The listing builds one solid part. Answer for the finished solid, in the listing's coordinates (mm). Round coordinates to 2 decimals unless told otherwise and drop trailing zeros. Loops run counter-clockwise (first coordinate to the right, second up) from the corner with the lowest first, then second, coordinate; pieces in that order, holes last. Notation, with made-up numbers: (84.25, -12) -> (93.25, -12) arc R13 ccw to (93.25, -7) -> close; hole circle Ø2 at (76.25, 71). An arc over 180 degrees is marked (long way). One line per question, with ' | ' between items.
from build123d import *

# Parameters (mm, degrees)
SKETCH1_R           = 5.56895
BOSS_EXTRUDE1_DEPTH = 23.8125
SKETCH2_R           = 1.5875
BOSS_EXTRUDE2_DEPTH = 3.175


with BuildPart() as part:
    # Sketch1 → Boss-Extrude1 (new, symmetric)
    with BuildSketch(Plane(origin=(0, 0, 0), x_dir=(0, 0, -1), z_dir=(1, 0, 0))):
        Circle(SKETCH1_R)
    extrude(amount=BOSS_EXTRUDE1_DEPTH, both=True)

    # Sketch2 → Boss-Extrude2 (add)
    with BuildSketch(Plane.ZY.offset(23.8125)):
        Circle(SKETCH2_R)
    boss_extrude2 = extrude(amount=BOSS_EXTRUDE2_DEPTH)

    # Sketch5 → Revolve1 (revolve)
    with BuildSketch(Plane.XY):
        with BuildLine():
            Line((-35.1917, 0), (-26.3525, 0))
            ThreePointArc((-26.3525, 0), (-30.7721, 4.4196), (-35.1917, 0))
        make_face()
    revolve1 = revolve(axis=Axis((-35.1917, 0, 0), (1, 0, 0)))

    # Mirror2: Boss-Extrude2, Revolve1 across plane
    add(boss_extrude2.mirror(Plane(origin=(0, 0, 0), x_dir=(0, 0, 1), z_dir=(1, 0, 0))))
    add(revolve1.mirror(Plane(origin=(0, 0, 0), x_dir=(0, 0, 1), z_dir=(1, 0, 0))))


solid = part.part
Q1. For a pull along X with two mould halves and no side action, classify faces 1 (the face through (0.333, 5.522, 0.725)), 2 (the face through (-23.812, 1.3, -1.2)), 3 (the face through (25.21, 0.477, 1.514)) as pulls with the +X half, pulls with the -X half, needs draft (parallel to the pull), parting line crosses it, or undercut.
Numbers:
face 1: needs draft | face 2: undercut | face 3: undercut
Q2. A cutting plane is placed at A-A on y = 0. Give the vertices of the cut face in (x, z).
Numbers:
outline: (-26.65, -1.59) -> (-23.81, -1.59) -> (-23.81, -5.57) -> (23.81, -5.57) -> (23.81, -1.59) -> (26.65, -1.59) arc R4.42 ccw (long way) to (26.65, 1.59) -> (23.81, 1.59) -> (23.81, 5.57) -> (-23.81, 5.57) -> (-23.81, 1.59) -> (-26.65, 1.59) arc R4.42 ccw (long way) to start
Q3. Given pin 1 Ø1 at (y, z) = (4.5, -3.5) entering from -X; pin 2 Ø2 at (x, z) = (10, 3.5) entering from -Y; pin 3 Ø2 at (x, y) = (-25.5, -0.5) entering from +Z, each flat-ended and moving along its own axis, determine where each tip first touches the part or whether it passes through.
Numbers:
pin 1: x = -23.81 | pin 2: y = -4.98 | pin 3: z = 1.59
Q4. Find the intervals of material crossed by line 1 (X direction, y = -2.5, z = 0.5); line 2 (X direction, y = -2.75, z = 1.25); line 3 (X direction, y = 3.75, z = -3.5), in increasing order. Write a range as from..to.
Numbers:
line 1: -34.38..-27.16, -23.81..23.81, 27.16..34.38 | line 2: -34..-27.55, -23.81..23.81, 27.55..34 | line 3: -23.81..23.81
Q5. A cutting plane is placed at C-C on x = -14.5. Give the vertices of the cut face in (y, z).
Numbers:
outline: circle Ø11.14 at (0, 0)
Q6. A cutting plane is placed at D-D on y = 3.5. Give the vertices of the cut face in (x, z), plus the area to 3 significant figures.
Numbers:
outline: circle Ø5.4 at (-30.77, 0); (-23.81, -4.33) -> (23.81, -4.33) -> (23.81, 4.33) -> (-23.81, 4.33) -> close; circle Ø5.4 at (30.77, 0) | area: 458 mm^2
